For this review, take the finished solid that the model builds, in its own axes (mm). Round coordinates to 2 decimals unless told otherwise and drop trailing zeros. Write each loop counter-clockwise with the first axis right and the second up, starting at its lowest first coordinate (ties: lowest second). Pieces come first, ordered by that corner, then holes. Notation, with made-up numbers: (16, 86.5) - (57, 86.5) arc R22 ccw to (57, 114.5) - close; hole circle Ø3 at (67.5, -37.75). An arc over 180 degrees is marked (long way). One line per item, written item: value. Start each with the question number.
Q1. For probe 1 along X at (y, z) = (16, 24.75); probe 2 along Y at (x, z) = (10.5, 15.25); probe 3 along Y at (x, z) = (13, 3.5), list the stretches that pass through material, from the lowest coordinate up.
Q2. Add section A-A on z = 15.25. Write out the cut boundary in (x, y), and give its area (3 significant figures).
Q3. Add section C-C on y = -15. Write out the cut boundary in (x, z).
Q4. Clearance check with a flat-ended pin moving along its axis: pin 1 Ø12 at (y, z) = (13.5, 4.5) entering from +X. State where the tip first meets the part, or that it passes through.
Q5. Add section B-B on x = -9. Write out the cut boundary in (y, z).
```python
from build123d import *

# Parameters (mm, degrees)
F1_DEPTH = 25.4
F3_DEPTH = 25.4


with BuildPart() as f1:
    # F0 (on Top) → F1 (new body)
    with BuildSketch(Plane.XY):
        Polygon((17.57632, -7.28035), (17.57632, 7.28035), (7.28035, 17.57632), (-7.28035, 17.57632), (-17.57632, 7.28035), (-17.57632, -7.28035), (-7.28035, -17.57632), (7.28035, -17.57632), align=None)
    extrude(amount=F1_DEPTH)

    # F2 (on Top) → F3 (join)
    with BuildSketch(Plane.XY):
        Polygon((14.142192, -0.699994), (9.36479, 10.620372), (-2.46449, 13.943381), (-12.437959, 6.76674), (-13.045391, -5.505394), (-3.829378, -13.631854), (8.270235, -11.49325), align=None)
    extrude(amount=F3_DEPTH)


solid = f1.part
```
Result set:
1. probe 1: x = -8.86 to 8.86
1. probe 2: y = -14.36 to 14.36
1. probe 3: y = -11.86 to 11.86
2. outline: (-17.58, -7.28) - (-7.28, -17.58) - (7.28, -17.58) - (17.58, -7.28) - (17.58, 7.28) - (7.28, 17.58) - (-7.28, 17.58) - (-17.58, 7.28) - close
2. area: 1,020 mm^2
3. outline: (-9.86, 0) - (9.86, 0) - (9.86, 25.4) - (-9.86, 25.4) - close
4. pin 1: stops at x = 17.36
5. outline: (-15.86, 0) - (15.86, 0) - (15.86, 25.4) - (-15.86, 25.4) - close
